CAD build for the part. Positions are in the model's coordinates, mm. A direction names the side the tool comes from. Give positions to 0.01 mm unless a question says otherwise; leave off trailing zeros. Write each loop counter-clockwise with the first axis right and the second up, starting at its lowest first coordinate (ties: lowest second). Pieces come first, ordered by that corner, then holes. Notation, with made-up numbers: (64.5, 9) -> (69.5, 9) arc R36 cw to (69.5, 44) -> close; hole circle Ø4 at (38.25, 31). An arc over 180 degrees is marked (long way). Answer as a JSON object with one key per item and string values.
```python
from build123d import *

# Parameters (mm, degrees)
F0_W     = 50.8
F0_H     = 50.8
F1_DEPTH = 50.8
F3_DEPTH = 38.1
F4_W     = 12.973598972
F4_H     = 12.9839326696
F5_DEPTH = 38.1
F6_DEPTH = 12.7
F7_DEPTH = 12.7


with BuildPart() as f1:
    # F0 (on Front) → F1 (new body)
    with BuildSketch(Plane.XZ):
        with Locations((-18.5270585775, 7.0019777209)):
            Rectangle(F0_W, F0_H)
    extrude(amount=F1_DEPTH)

    # F2 (on face) → F3 (cut)
    with BuildSketch(Plane.XZ.offset(50.8)):
        Polygon((6.8729414225, 32.4019777209), (6.8729414225, 17.4989413492), (25.4, 17.4989413492), (25.4, 42.8989413492), (0, 42.8989413492), (0, 32.4019777209), align=None)
    extrude(amount=-F3_DEPTH, mode=Mode.SUBTRACT)

    # F4 (on face) → F5 (cut)
    with BuildSketch(Plane.YZ.offset(6.8729414225)):
        with Locations((-44.313200514, 25.910011386)):
            Rectangle(F4_W, F4_H)
    extrude(amount=-F5_DEPTH, mode=Mode.SUBTRACT)

    # F6 (add): a face of the model
    f6_faces = [f1.faces().sort_by_distance(p)[0] for p in [
        (-12.1770585775, -37.826401028, 25.910011386),
    ]]
    extrude(f6_faces, amount=-F6_DEPTH)

    # F7 (cut): a face of the model
    f7_faces = [f1.faces().sort_by_distance(p)[0] for p in [
        (-12.1770585775, -37.826401028, 25.910011386),
    ]]
    extrude(f7_faces, amount=-F7_DEPTH, mode=Mode.SUBTRACT)


solid = f1.part
```
1) Slice it at A-A (x = -26.5). List the corners of the cut face in (y, z), then the cut area to 3 significant figures.
Model answer:
{"outline": "(-50.8, -18.4) -> (0, -18.4) -> (0, 32.4) -> (-25.13, 32.4) -> (-25.13, 19.42) -> (-50.8, 19.42) -> close", "area": "2,250 mm2"}
2) Slice it at B-B (y = -38). List the corners of the cut face in (x, z).
Model answer:
{"outline": "(-43.93, -18.4) -> (6.87, -18.4) -> (6.87, 19.42) -> (-31.23, 19.42) -> (-31.23, 32.4) -> (-43.93, 32.4) -> close"}
3) 3-axis set-ups, long thin cutter, end or side, ignore diameter. For faces 1 (the flat face through (-19, -50.8, 2)), 2 (the flat face through (-12, -25.126, 26)): which of +Z, -Z, +X, -X, +Y, -Y reach the whole face in a straight line?
Model answer:
{"face 1": "+Z, -Z, +X, -X, -Y", "face 2": "+Z, +X, -Y"}
4) Wall check: probe 1 along Y at (x, z) = (-1.5, 21); probe 2 along X at (y, z) = (-40, 25); probe 3 along Z at (x, y) = (-21.5, -29). Give the ranges that are in metal, low to high.
Model answer:
{"probe 1": "y = -25.13 to 0", "probe 2": "x = -43.93 to -31.23", "probe 3": "z = -18.4 to 19.42"}
5) Pin check, flat tips, straight feed: pin 1 (10.5 mm diameter, centred on x = -16.5, z = 26.5, fed in from -Y); pin 2 (10 mm diameter, centred on x = -11.5, y = -37, fed in from +Z); pin 3 (10.5 mm diameter, centred on y = -32.5, z = 25.5, fed in from +X). Stop position of each tip, or through.
Model answer:
{"pin 1": "stops at y = -25.13", "pin 2": "stops at z = 19.42", "pin 3": "stops at x = -31.23"}
